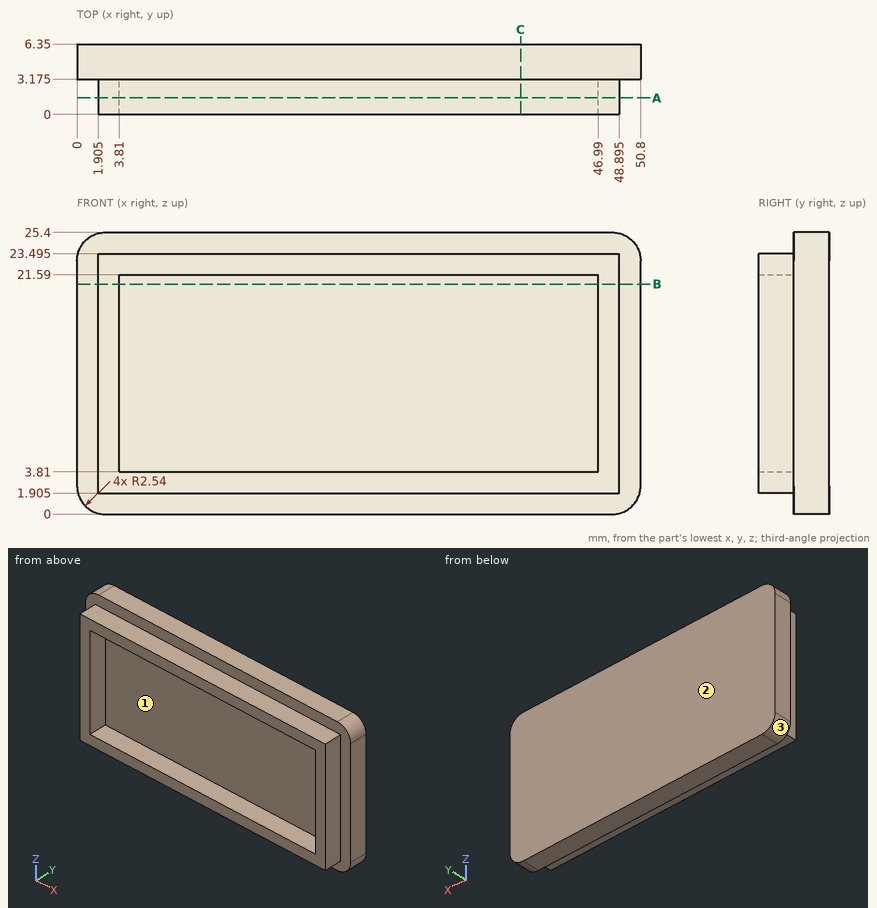
Design review of the part shown in the three views and the two pictorial views. Dimensions are in mm from the part's minimum x, y and z. Round coordinates to 2 decimals unless told otherwise and drop trailing zeros. Loops run counter-clockwise (first coordinate to the right, second up) from the corner with the lowest first, then second, coordinate; pieces in that order, holes last. Notation, with made-up numbers: (84, 4.25) - (124, 4.25) arc R24 ccw to (124, 34.25) - close; hole circle Ø1 at (86.5, -18.75). An arc over 180 degrees is marked (long way). Use CSV: the item, a comma, the result in double quotes.
(1) Clearance check with flat-ended pins moving along their axes: P1, Ø3, axis at y = 1.5, z = 20, coming from the +X side (3 decimals); P2, Ø1.6, axis at y = 1, z = 9.5, coming from the -X side (3 decimals); P3, Ø1, axis at x = 15.5, y = 1, coming from the -Z side (3 decimals). State where each tip first meets the part, or that it passes through.
Working result:
P1,"stops at x = 48.895"
P2,"stops at x = 1.905"
P3,"stops at z = 1.905"
(2) Take a section at C-C, the plane x = 40. Give the boundary of the cut face in (y, z) (3 decimals), plus the area to 3 significant figures.
Working result:
outline,"(0, 1.905) - (3.175, 1.905) - (3.175, 0) - (6.35, 0) - (6.35, 25.4) - (3.175, 25.4) - (3.175, 23.495) - (0, 23.495) - (0, 21.59) - (3.175, 21.59) - (3.175, 3.81) - (0, 3.81) - close"
area,"92.7 mm^2"
(3) For line 1 (Z direction, x = 32, y = 2.5) (3 decimals); line 2 (X direction, y = 0.5, z = 20.5) (3 decimals); line 3 (Y direction, x = 29.5, z = 16.25) (3 decimals), list the stretches that pass through material, from the lowest coordinate up.
Working result:
line 1,"z = 1.905 to 3.81, 21.59 to 23.495"
line 2,"x = 1.905 to 3.81, 46.99 to 48.895"
line 3,"y = 3.175 to 6.35"
(4) Take a section at B-B, the plane z = 20.75. Give the boundary of the cut face in (x, y) (3 decimals).
Working result:
outline,"(0, 3.175) - (1.905, 3.175) - (1.905, 0) - (3.81, 0) - (3.81, 3.175) - (46.99, 3.175) - (46.99, 0) - (48.895, 0) - (48.895, 3.175) - (50.8, 3.175) - (50.8, 6.35) - (0, 6.35) - close"
(5) The part is to be moulded in two halves that separate along Z. For the marked faces 1, 2 and 3, say which applies: pulls with the +Z half, pulls with the -Z half, needs draft (parallel to the pull), parting line crosses it, or undercut.
Working result:
face 1,"undercut"
face 2,"needs draft"
face 3,"pulls with the -Z half"
(6) Take a section at A-A, the plane y = 1.5. Give the boundary of the cut face in (x, z) (3 decimals), plus the area to 3 significant figures.
Working result:
outline,"(1.905, 1.905) - (48.895, 1.905) - (48.895, 23.495) - (1.905, 23.495) - close; hole (3.81, 3.81) - (46.99, 3.81) - (46.99, 21.59) - (3.81, 21.59) - close"
area,"247 mm^2"
